from build123d import *

# Parameters (mm, degrees)
SKETCH_1_R          = 87.5
EXTRUDE_1_DEPTH     = 16
CUT_EXTRUDE_1_REACH = 186.543
SKETCH_2_R          = 5.15


with BuildPart() as part:
    # 草图1 → 凸台-拉伸1 (new body)
    with BuildSketch(Plane.XY):
        with BuildLine():
            Line((-130, 0), (-130, -125))
            Line((-130, -125), (130, -125))
            Line((130, -125), (130, 0))
            ThreePointArc((130, 0), (0, 130), (-130, 0))
        make_face()
        Circle(SKETCH_1_R, mode=Mode.SUBTRACT)
    extrude(amount=EXTRUDE_1_DEPTH)

    # 草图2 → 切除-拉伸1 (cut, up to next)
    with BuildSketch(Plane.XY.offset(16), mode=Mode.PRIVATE) as cut_extrude_1_sk1:
        with Locations((-26.528952123, 99.007397195)):
            Circle(SKETCH_2_R)
    cut_extrude_1_tool1 = extrude(cut_extrude_1_sk1.sketch, amount=-CUT_EXTRUDE_1_REACH, mode=Mode.PRIVATE) & part.part
    # 草图2 → 切除-拉伸1 (cut, up to next)
    with BuildSketch(Plane.XY.offset(16), mode=Mode.PRIVATE) as cut_extrude_1_sk2:
        with Locations((26.528952123, 99.007397195)):
            Circle(SKETCH_2_R)
    cut_extrude_1_tool2 = extrude(cut_extrude_1_sk2.sketch, amount=-CUT_EXTRUDE_1_REACH, mode=Mode.PRIVATE) & part.part
    # 草图2 → 切除-拉伸1 (cut, up to next)
    with BuildSketch(Plane.XY.offset(16), mode=Mode.PRIVATE) as cut_extrude_1_sk3:
        with Locations((72.478445072, 72.478445072)):
            Circle(SKETCH_2_R)
    cut_extrude_1_tool3 = extrude(cut_extrude_1_sk3.sketch, amount=-CUT_EXTRUDE_1_REACH, mode=Mode.PRIVATE) & part.part
    # 草图2 → 切除-拉伸1 (cut, up to next)
    with BuildSketch(Plane.XY.offset(16), mode=Mode.PRIVATE) as cut_extrude_1_sk4:
        with Locations((99.007397195, 26.528952123)):
            Circle(SKETCH_2_R)
    cut_extrude_1_tool4 = extrude(cut_extrude_1_sk4.sketch, amount=-CUT_EXTRUDE_1_REACH, mode=Mode.PRIVATE) & part.part
    # 草图2 → 切除-拉伸1 (cut, up to next)
    with BuildSketch(Plane.XY.offset(16), mode=Mode.PRIVATE) as cut_extrude_1_sk5:
        with Locations((99.007397195, -26.528952123)):
            Circle(SKETCH_2_R)
    cut_extrude_1_tool5 = extrude(cut_extrude_1_sk5.sketch, amount=-CUT_EXTRUDE_1_REACH, mode=Mode.PRIVATE) & part.part
    # 草图2 → 切除-拉伸1 (cut, up to next)
    with BuildSketch(Plane.XY.offset(16), mode=Mode.PRIVATE) as cut_extrude_1_sk6:
        with Locations((72.478445072, -72.478445072)):
            Circle(SKETCH_2_R)
    cut_extrude_1_tool6 = extrude(cut_extrude_1_sk6.sketch, amount=-CUT_EXTRUDE_1_REACH, mode=Mode.PRIVATE) & part.part
    # 草图2 → 切除-拉伸1 (cut, up to next)
    with BuildSketch(Plane.XY.offset(16), mode=Mode.PRIVATE) as cut_extrude_1_sk7:
        with Locations((26.528952123, -99.007397195)):
            Circle(SKETCH_2_R)
    cut_extrude_1_tool7 = extrude(cut_extrude_1_sk7.sketch, amount=-CUT_EXTRUDE_1_REACH, mode=Mode.PRIVATE) & part.part
    # 草图2 → 切除-拉伸1 (cut, up to next)
    with BuildSketch(Plane.XY.offset(16), mode=Mode.PRIVATE) as cut_extrude_1_sk8:
        with Locations((-26.528952123, -99.007397195)):
            Circle(SKETCH_2_R)
    cut_extrude_1_tool8 = extrude(cut_extrude_1_sk8.sketch, amount=-CUT_EXTRUDE_1_REACH, mode=Mode.PRIVATE) & part.part
    # 草图2 → 切除-拉伸1 (cut, up to next)
    with BuildSketch(Plane.XY.offset(16), mode=Mode.PRIVATE) as cut_extrude_1_sk9:
        with Locations((-72.478445072, -72.478445072)):
            Circle(SKETCH_2_R)
    cut_extrude_1_tool9 = extrude(cut_extrude_1_sk9.sketch, amount=-CUT_EXTRUDE_1_REACH, mode=Mode.PRIVATE) & part.part
    # 草图2 → 切除-拉伸1 (cut, up to next)
    with BuildSketch(Plane.XY.offset(16), mode=Mode.PRIVATE) as cut_extrude_1_sk10:
        with Locations((-99.007397195, -26.528952123)):
            Circle(SKETCH_2_R)
    cut_extrude_1_tool10 = extrude(cut_extrude_1_sk10.sketch, amount=-CUT_EXTRUDE_1_REACH, mode=Mode.PRIVATE) & part.part
    # 草图2 → 切除-拉伸1 (cut, up to next)
    with BuildSketch(Plane.XY.offset(16), mode=Mode.PRIVATE) as cut_extrude_1_sk11:
        with Locations((-99.007397195, 26.528952123)):
            Circle(SKETCH_2_R)
    cut_extrude_1_tool11 = extrude(cut_extrude_1_sk11.sketch, amount=-CUT_EXTRUDE_1_REACH, mode=Mode.PRIVATE) & part.part
    # 草图2 → 切除-拉伸1 (cut, up to next)
    with BuildSketch(Plane.XY.offset(16), mode=Mode.PRIVATE) as cut_extrude_1_sk12:
        with Locations((-72.478445072, 72.478445072)):
            Circle(SKETCH_2_R)
    cut_extrude_1_tool12 = extrude(cut_extrude_1_sk12.sketch, amount=-CUT_EXTRUDE_1_REACH, mode=Mode.PRIVATE) & part.part
    add(cut_extrude_1_tool1.solids().sort_by_distance((-26.528952, 99.007397, 16))[0], mode=Mode.SUBTRACT)
    add(cut_extrude_1_tool2.solids().sort_by_distance((26.528952, 99.007397, 16))[0], mode=Mode.SUBTRACT)
    add(cut_extrude_1_tool3.solids().sort_by_distance((72.478445, 72.478445, 16))[0], mode=Mode.SUBTRACT)
    add(cut_extrude_1_tool4.solids().sort_by_distance((99.007397, 26.528952, 16))[0], mode=Mode.SUBTRACT)
    add(cut_extrude_1_tool5.solids().sort_by_distance((99.007397, -26.528952, 16))[0], mode=Mode.SUBTRACT)
    add(cut_extrude_1_tool6.solids().sort_by_distance((72.478445, -72.478445, 16))[0], mode=Mode.SUBTRACT)
    add(cut_extrude_1_tool7.solids().sort_by_distance((26.528952, -99.007397, 16))[0], mode=Mode.SUBTRACT)
    add(cut_extrude_1_tool8.solids().sort_by_distance((-26.528952, -99.007397, 16))[0], mode=Mode.SUBTRACT)
    add(cut_extrude_1_tool9.solids().sort_by_distance((-72.478445, -72.478445, 16))[0], mode=Mode.SUBTRACT)
    add(cut_extrude_1_tool10.solids().sort_by_distance((-99.007397, -26.528952, 16))[0], mode=Mode.SUBTRACT)
    add(cut_extrude_1_tool11.solids().sort_by_distance((-99.007397, 26.528952, 16))[0], mode=Mode.SUBTRACT)
    add(cut_extrude_1_tool12.solids().sort_by_distance((-72.478445, 72.478445, 16))[0], mode=Mode.SUBTRACT)


solid = part.part
Work out the finished part from the listing and answer in its coordinate system (mm). Round coordinates to 2 decimals unless told otherwise and drop trailing zeros. Loops run counter-clockwise (first coordinate to the right, second up) from the corner with the lowest first, then second, coordinate; pieces in that order, holes last. Notation, with made-up numbers: (77, 45) - (128, 45) arc R25 ccw to (128, 65) - close; hole circle Ø11 at (19, -15.75). An arc over 180 degrees is marked (long way). Use one line per item in the form item = value. Start each with the question number.
(1) Determine the mould class of faces 1 (the face through (-64.49, 59.14, 7.89)), 2 (the face through (130, -63, 8)), 3 (the face through (-2, -125, 8)), 4 (the face through (2.86, 129.97, 7.89)) for opening direction Y: +Y half, -Y half, draft (parallel to the pull), parting line (faces both ways), or undercut.
(2) Find section C-C on z = 10.5. Give the number of separate pieces and of enclosed holes in the cut face, and give its area (3 significant figures).
(3) Find section B-B on x = 0. Determine the outline of the cut face in (y, z).
(4) Flat-ended cylindrical pins translate along their axes: P1, Ø3, axis at x = -29, z = 5, coming from the +Y side; P2, Ø13.5, axis at x = 99.01, y = -26.53, coming from the +Z side; P3, Ø5, axis at y = 99, z = 7, coming from the +X side; P4, Ø2, axis at x = -42.5, z = 11, coming from the +Y side. Find the tip coordinate at first contact, or state that the pin passes through.
(5) Find section D-D on y = 111. Determine the outline of the cut face in (x, z).
(6) Consider line 1 (X direction, y = 2, z = 5); line 2 (Y direction, x = -26, z = 1.75); line 3 (X direction, y = -97, z = 11). Determine where each line is inside the solid, lowest interval first.
(7) Find section A-A on y = -46.5. Determine the outline of the cut face in (x, z), and give its area (3 significant figures).
Answer list:
q1.face_1 = undercut
q1.face_2 = draft
q1.face_3 = -Y half
q1.face_4 = +Y half
q2.separate_pieces = 1
q2.enclosed_holes = 13
q2.area = 34,000 mm^2
q3.outline = (-125, 0) - (-87.5, 0) - (-87.5, 16) - (-125, 16) - close; (87.5, 0) - (130, 0) - (130, 16) - (87.5, 16) - close
q4.P1 = 127.06
q4.P2 = 16
q4.P3 = 87.11
q4.P4 = 123.2
q5.outline = (-67.67, 0) - (67.67, 0) - (67.67, 16) - (-67.67, 16) - close
q6.line_1 = -129.98 to -87.48, 87.48 to 129.98
q6.line_2 = -125 to -104.13, -93.88 to -83.55, 83.55 to 93.88, 104.13 to 127.37
q6.line_3 = -130 to -31.27, -21.79 to 21.79, 31.27 to 130
q7.outline = (-130, 0) - (-74.12, 0) - (-74.12, 16) - (-130, 16) - close; (74.12, 0) - (130, 0) - (130, 16) - (74.12, 16) - close
q7.area = 1,790 mm^2
